For this review, use the dimensioned drawing (mm, ordinates from the lowest corner) and the shaded views. A direction names the side the tool comes from. Round coordinates to 2 decimals unless told otherwise and drop trailing zeros. Order: outer loops, then holes, each group sorted by start corner. A loop starts at its lowest first (then second) coordinate and runs counter-clockwise, first axis right, second up. Notation, with made-up numbers: (15, 73.25) - (61, 73.25) arc R26 cw to (61, 95.25) - close; hole circle Ø10 at (70.25, 5). An arc over 180 degrees is marked (long way). Write item = value, one per line.
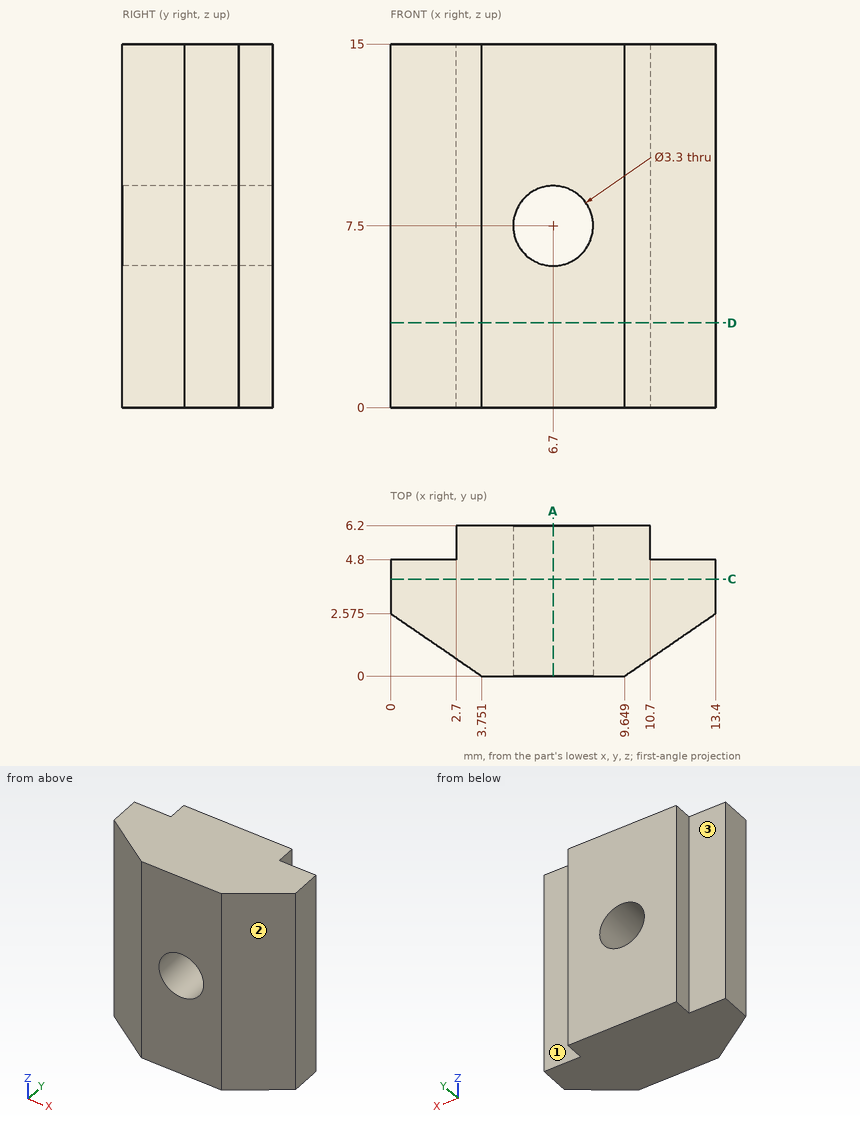
1) We need section A-A on x = 6.7. Write out the cut boundary in (y, z).
Findings:
outline = (0, 0) - (6.2, 0) - (6.2, 5.85) - (0, 5.85) - close; (0, 9.15) - (6.2, 9.15) - (6.2, 15) - (0, 15) - close
2) We need section C-C on y = 4. Write out the cut boundary in (x, z).
Findings:
outline = (0, 0) - (13.4, 0) - (13.4, 15) - (0, 15) - close; hole circle Ø3.3 at (6.7, 7.5)
3) To check wall thickness, follow L1, parallel to X at y = 4.25, z = 7.5; L2, parallel to X at y = 4.5, z = 8.5; L3, parallel to Y at x = 2.25, z = 3.75. State the ranges of each line that lie inside material, in increasing order. Write a range as from..to.
Findings:
L1 = 0..5.05, 8.35..13.4
L2 = 0..5.39, 8.01..13.4
L3 = 1.03..4.8
4) Clearance check with flat-ended pins moving along their axes: pin 1 Ø1.4 at (x, z) = (1.5, 8) entering from +Y; pin 2 Ø1 at (x, y) = (11.5, 2) entering from -Z; pin 3 Ø1.1 at (y, z) = (5.5, 8.5) entering from -X. State where each tip first meets the part, or that it passes through.
Findings:
pin_1 = 4.8
pin_2 = 0
pin_3 = 2.7
5) We need section D-D on z = 3.5. Write out the cut boundary in (x, y) (1 decimal).
Findings:
outline = (0, 2.6) - (3.8, 0) - (9.6, 0) - (13.4, 2.6) - (13.4, 4.8) - (10.7, 4.8) - (10.7, 6.2) - (2.7, 6.2) - (2.7, 4.8) - (0, 4.8) - close
6) For the marked faces 1, 2 and 3, list the 3-axis set-ups (+Z, -Z, +X, -X, +Y, -Y) from which the entire face can be reached by the end or side of a thin tool; tool diameter is ignored.
Findings:
face_1 = +Z, -Z, +X, +Y
face_2 = +Z, -Z, +X, -Y
face_3 = +Z, -Z, -X, +Y
